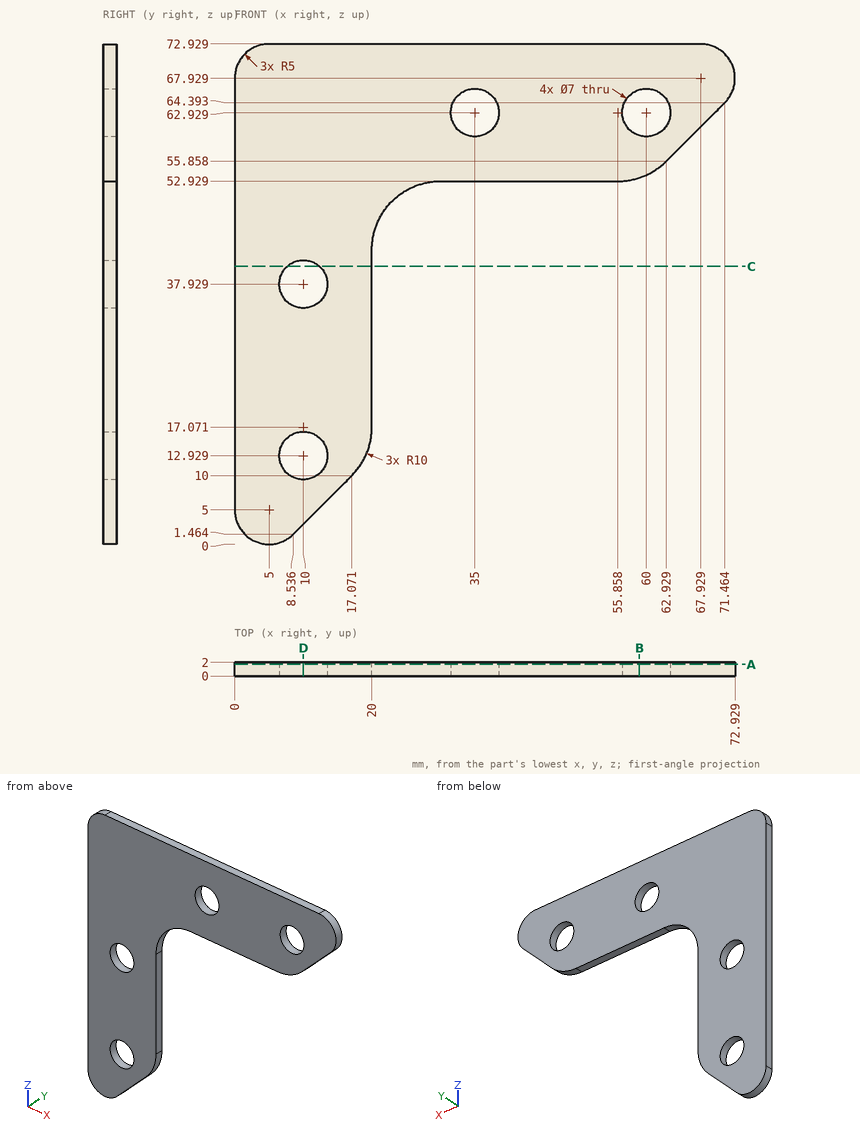
Input: dimensioned drawing with shaded views. Units: mm. Origin: part minimum x, y, z. Give positions to 0.01 mm unless a question says otherwise; leave off trailing zeros. Order: outer loops, then holes, each group sorted by start corner. A loop starts at its lowest first (then second) coordinate and runs counter-clockwise, first axis right, second up.
(1) Section query B-B (x = 59). Return the cut outline in (y, z) (1 decimal).
(2) Section query A-A (y = 1.7). Return the cut outline in (x, z) (1 decimal).
(3) Material intervals for line 1 along X through (y, z) = (1.4, 62) (1 decimal); line 2 along Z through (x, y) = (45, 0.5); line 3 along X through (y, z) = (0.7, 10.5), sorted ascending.
(4) Section query C-C (z = 40.5). Return the cut outline in (x, y) (1 decimal).
(5) Section query D-D (x = 10). Return the cut outline in (y, z).
Outcome:
1. outline: (0, 53.4) - (2, 53.4) - (2, 59.6) - (0, 59.6) - close; (0, 66.3) - (2, 66.3) - (2, 72.9) - (0, 72.9) - close
2. outline: (0, 5) arc R5 ccw to (8.5, 1.5) - (17.1, 10) arc R10 ccw to (20, 17.1) - (20, 42.9) arc R10 cw to (30, 52.9) - (55.9, 52.9) arc R10 ccw to (62.9, 55.9) - (71.5, 64.4) arc R5 ccw to (67.9, 72.9) - (5, 72.9) arc R5 ccw to (0, 67.9) - close; hole circle Ø7 at (10, 12.9); hole circle Ø7 at (10, 37.9); hole circle Ø7 at (35, 62.9); hole circle Ø7 at (60, 62.9)
3. line 1: x = 0 to 31.6, 38.4 to 56.6, 63.4 to 69.1
3. line 2: z = 52.93 to 72.93
3. line 3: x = 0 to 7.48, 12.52 to 17.54
4. outline: (0, 0) - (7.6, 0) - (7.6, 2) - (0, 2) - close; (12.4, 0) - (20, 0) - (20, 2) - (12.4, 2) - close
5. outline: (0, 2.93) - (2, 2.93) - (2, 9.43) - (0, 9.43) - close; (0, 16.43) - (2, 16.43) - (2, 34.43) - (0, 34.43) - close; (0, 41.43) - (2, 41.43) - (2, 72.93) - (0, 72.93) - close
